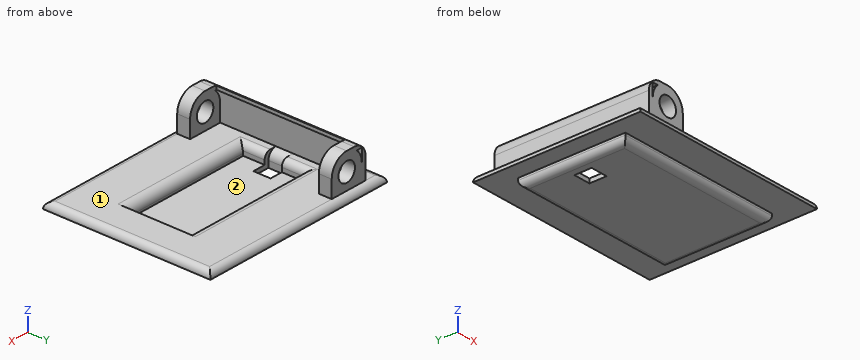
```python
from build123d import *

# Parameters (mm, degrees)
ESQUISSE1_W             = 47
ESQUISSE1_H             = 39
BOSS_EXTRU_1_DEPTH      = 2.5
ESQUISSE2_W             = 8
ESQUISSE2_H             = 3
BOSS_EXTRU_2_DEPTH      = 8
ESQUISSE3_R             = 2.192012696
ENL_V_MAT_EXTRU_1_DEPTH = 62.036874101
CONG_1_R                = 4
ESQUISSE4_W             = 31
ESQUISSE4_H             = 14
ENL_V_MAT_EXTRU_2_DEPTH = 20
CONG_2_R                = 2
ESQUISSE8_W             = 1
ESQUISSE8_H             = 36
BOSS_EXTRU_5_DEPTH      = 8
ESQUISSE9_W             = 1
ESQUISSE9_H             = 36
BOSS_EXTRU_6_DEPTH      = 4
ESQUISSE10_W            = 7.449336574
ESQUISSE10_H            = 30
ENL_V_MAT_EXTRU_4_DEPTH = 8
CONG_4_R                = 3
ESQUISSE11_OUTSIDE_W    = 61.394
ESQUISSE11_OUTSIDE_H    = 53.394
ESQUISSE11_OUTSIDE_W_2  = 39
ESQUISSE11_OUTSIDE_H_2  = 25
ENL_V_MAT_EXTRU_5_DEPTH = 1
ESQUISSE12_W            = 39
ESQUISSE12_H            = 25
BOSS_EXTRU_7_DEPTH      = 1
ENL_V_MAT_EXTRU_6_REACH = 63.595
ESQUISSE13_W            = 4
ESQUISSE13_H            = 4
CONG_6_R                = 2
CONG_7_R                = 1.5
CONG_8_R                = 1.5


# Some blends are built 0.0001 mm under size
with BuildPart() as part:
    # Esquisse1 → Boss.-Extru.1 (new body)
    with BuildSketch(Plane.XY):
        with Locations((23.5, 19.5)):
            Rectangle(ESQUISSE1_W, ESQUISSE1_H)
    extrude(amount=BOSS_EXTRU_1_DEPTH)

    # Esquisse2 → Boss.-Extru.2 (add)
    with BuildSketch(Plane.XY.offset(2.5)):
        with Locations((9, 36)):
            Rectangle(ESQUISSE2_W, ESQUISSE2_H)
        with Locations((9, 3)):
            Rectangle(ESQUISSE2_W, ESQUISSE2_H)
    extrude(amount=BOSS_EXTRU_2_DEPTH)

    # Esquisse3 → Enlèv. mat.-Extru.1 (cut, through all)
    with BuildSketch(Plane.XZ.offset(-1.5)):
        with Locations(Location((9, 6.3, 0), (0, 0, 270))):
            Circle(ESQUISSE3_R)
    extrude(amount=-ENL_V_MAT_EXTRU_1_DEPTH, mode=Mode.SUBTRACT)

    # Congé1
    cong_1_edges = [part.edges().sort_by_distance(p)[0] for p in [
        (13, 3, 10.5),
        (5, 3, 10.5),
        (13, 36, 10.5),
        (5, 36, 10.5),
    ]]
    fillet(cong_1_edges, radius=CONG_1_R - 0.0001)  # a hair under: the kernel refuses the full size

    # Esquisse4 → Enlèv. mat.-Extru.2 (cut)
    with BuildSketch(Plane.XY.offset(2.5)):
        with Locations((23.5, 19.5)):
            Rectangle(ESQUISSE4_W, ESQUISSE4_H)
    extrude(amount=-ENL_V_MAT_EXTRU_2_DEPTH, mode=Mode.SUBTRACT)

    # Congé2
    cong_2_edges = [part.edges().sort_by_distance(p)[0] for p in [
        (23.5, 12.5, 2.5),
        (23.5, 26.5, 2.5),
    ]]
    fillet(cong_2_edges, radius=CONG_2_R)

    # Esquisse8 → Boss.-Extru.5 (add)
    with BuildSketch(Plane.XY.offset(2.5)):
        with Locations((4.5, 19.5)):
            Rectangle(ESQUISSE8_W, ESQUISSE8_H)
    extrude(amount=BOSS_EXTRU_5_DEPTH)

    # Esquisse9 → Boss.-Extru.6 (add)
    with BuildSketch(Plane(origin=(5, 0, 0), x_dir=(0, 0, -1), z_dir=(1, 0, 0))):
        with Locations((-10, 19.5)):
            Rectangle(ESQUISSE9_W, ESQUISSE9_H)
    extrude(amount=BOSS_EXTRU_6_DEPTH)

    # Esquisse10 → Enlèv. mat.-Extru.4 (cut)
    with BuildSketch(Plane.XY.offset(10.5)):
        with Locations((9.724668287, 19.5)):
            Rectangle(ESQUISSE10_W, ESQUISSE10_H)
    extrude(amount=-ENL_V_MAT_EXTRU_4_DEPTH, mode=Mode.SUBTRACT)

    # Congé4
    # the kernel refuses this fillet: 3 mm, written as the material it takes off along each edge
    with BuildSketch(Plane(origin=(4, -6, 10.5), x_dir=(1, 0, 0), z_dir=(0, 1, 0))) as cong_4_piece_1:
        with BuildLine():
            CenterArc((CONG_4_R, CONG_4_R), CONG_4_R, 180, 90)
            Line((0, CONG_4_R), (0, 0))
            Line((0, 0), (CONG_4_R, 0))
        make_face()
    extrude(amount=51, mode=Mode.SUBTRACT)

    # Esquisse11 outside → Enlèv. mat.-Extru.5 (cut)
    with BuildSketch(Plane(origin=(0, 0, 0), x_dir=(-1, 0, 0), z_dir=(0, 0, -1))):
        with Locations((-23.5, 19.5)):
            Rectangle(ESQUISSE11_OUTSIDE_W, ESQUISSE11_OUTSIDE_H)
        with Locations((-23.5, 19.5)):
            Rectangle(ESQUISSE11_OUTSIDE_W_2, ESQUISSE11_OUTSIDE_H_2, mode=Mode.SUBTRACT)
    extrude(amount=-ENL_V_MAT_EXTRU_5_DEPTH, mode=Mode.SUBTRACT)

    # Esquisse12 → Boss.-Extru.7 (add)
    with BuildSketch(Plane(origin=(0, 0, 0), x_dir=(-1, 0, 0), z_dir=(0, 0, -1))):
        with Locations((-23.5, 19.5)):
            Rectangle(ESQUISSE12_W, ESQUISSE12_H)
    extrude(amount=BOSS_EXTRU_7_DEPTH)

    # Esquisse13 → Enlèv. mat.-Extru.6 (cut, up to next)
    with BuildSketch(Plane.XY.offset(2.5), mode=Mode.PRIVATE) as enl_v_mat_extru_6_sk1:
        with Locations((9, 19.5)):
            Rectangle(ESQUISSE13_W, ESQUISSE13_H)
    enl_v_mat_extru_6_tool1 = extrude(enl_v_mat_extru_6_sk1.sketch, amount=-ENL_V_MAT_EXTRU_6_REACH, mode=Mode.PRIVATE) & part.part
    add(enl_v_mat_extru_6_tool1.solids().sort_by_distance((9, 19.5, 2.5))[0], mode=Mode.SUBTRACT)

    # Congé6
    cong_6_edges = [part.edges().sort_by_distance(p)[0] for p in [
        (7, 19.5, 2.5),
    ]]
    fillet(cong_6_edges, radius=CONG_6_R - 0.0001)  # a hair under: the kernel refuses the full size

    # Congé7
    cong_7_edges = [part.edges().sort_by_distance(p)[0] for p in [
        (8, 25, 2.5),
        (8, 14, 2.5),
        (0, 19.5, 2.5),
        (23.5, 0, 2.5),
        (47, 19.5, 2.5),
        (23.5, 39, 2.5),
    ]]
    fillet(cong_7_edges, radius=CONG_7_R - 0.0001)  # a hair under: the kernel refuses the full size

    # Congé8
    cong_8_edges = [part.edges().sort_by_distance(p)[0] for p in [
        (43, 19.5, -1),
        (23.5, 7, -1),
        (4, 19.5, -1),
        (23.5, 32, -1),
    ]]
    fillet(cong_8_edges, radius=CONG_8_R)


solid = part.part
```
Design review of the part built by this model. Coordinates are the model's own, in mm. Face numbers are marked on the shaded views. Give positions to 0.01 mm unless a question says otherwise; leave off trailing zeros. Order: outer loops, then holes, each group sorted by start corner. A loop starts at its lowest first (then second) coordinate and runs counter-clockwise, first axis right, second up. Notation, with made-up numbers: (85, 24) -> (138, 24) arc R24 ccw to (138, 37) -> close; hole circle Ø7 at (21.5, -34.5). An arc over 180 degrees is marked (long way). Write item = value, one per line. Start each with the question number.
(1) Mouldability with a two-part tool opening along X and no side actions: class the marked faces 1 and 2 as +X half, -X half, draft (parallel to the pull), parting line (faces both ways), or undercut.
(2) We need section B-B on z = 5.5. Write out the cut boundary in (x, y).
(3) To check wall thickness, follow line 1 along X through (y, z) = (3.7, 6.3); line 2 along X through (y, z) = (14, 4); line 3 along Z through (x, y) = (9.5, 29). State the ranges of each line that lie inside material, in increasing order.
(4) For pin 1 (11 mm diameter, centred on x = 17.5, y = 13, fed in from +Z); pin 2 (0.5 mm diameter, centred on y = 14, z = 0.5, fed in from +X); pin 3 (3 mm diameter, centred on x = 10.5, z = 8.5, fed in from +Y); pin 4 (2 mm diameter, centred on x = 17.5, z = 4, fed in from +Y), all flat-tipped, find the tip position at first contact; note any pin that passes through.
(5) We need section A-A on y = 4. State how many separate pieces and enclosed holes the cut face has, plus the area to 3 significant figures.
Numbers:
q1.face_1 = draft
q1.face_2 = undercut
q2.outline = (4, 1.5) -> (6.96, 1.5) -> (6.96, 4.5) -> (5, 4.5) -> (5, 34.5) -> (6.96, 34.5) -> (6.96, 37.5) -> (4, 37.5) -> close; (11.04, 1.5) -> (13, 1.5) -> (13, 4.5) -> (11.04, 4.5) -> close; (11.04, 34.5) -> (13, 34.5) -> (13, 37.5) -> (11.04, 37.5) -> close
q3.line_1 = 4 to 6.81, 11.19 to 13
q3.line_2 = 4 to 5
q3.line_3 = -1 to 2.5
q4.pin_1 = 2.5
q4.pin_2 = 43
q4.pin_3 = 37.5
q4.pin_4 = through
q5.separate_pieces = 1
q5.enclosed_holes = 2
q5.area = 120 mm^2
